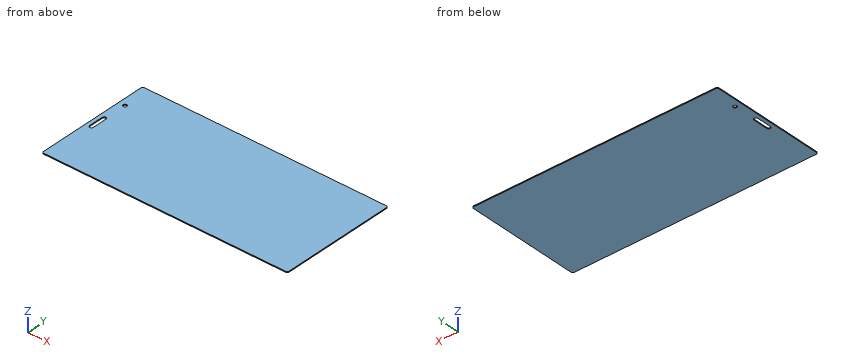
from build123d import *

# Parameters (mm, degrees)
CYLINDER010_R     = 1
CYLINDER010_DEPTH = 10
BOX016_W          = 2
BOX016_H          = 10
BOX016_DEPTH      = 10
FILLET008_R       = 0.95
BOX004_W          = 133
BOX004_H          = 63
BOX004_DEPTH      = 0.5
FILLET005_R       = 1


with BuildPart() as cilindro010:
    # Cylinder010 → Cylinder010 (new body)
    with BuildSketch(Plane(origin=(5.5, 50, 0), x_dir=(1, 0, 0), z_dir=(0, 0, 1))):
        Circle(CYLINDER010_R)
    extrude(amount=CYLINDER010_DEPTH)


with BuildPart() as fillet008:
    # Box016 → Box016 (new body)
    with BuildSketch(Plane(origin=(4, 28.5, 0), x_dir=(1, 0, 0), z_dir=(0, 0, 1))):
        with Locations((1, 5)):
            Rectangle(BOX016_W, BOX016_H)
    extrude(amount=BOX016_DEPTH)

    # Fillet008
    fillet008_edges = [fillet008.edges().sort_by_distance(p)[0] for p in [
        (4, 28.5, 5),
        (4, 38.5, 5),
        (6, 28.5, 5),
        (6, 38.5, 5),
    ]]
    fillet(fillet008_edges, radius=FILLET008_R)


with BuildPart() as cut016:
    # Box004 → Box004 (new body)
    with BuildSketch(Plane(origin=(2, 2, 5.5), x_dir=(1, 0, 0), z_dir=(0, 0, 1))):
        with Locations((66.5, 31.5)):
            Rectangle(BOX004_W, BOX004_H)
    extrude(amount=BOX004_DEPTH)

    # Fillet005
    fillet005_edges = [cut016.edges().sort_by_distance(p)[0] for p in [
        (2, 2, 5.75),
        (2, 65, 5.75),
        (135, 2, 5.75),
        (135, 65, 5.75),
    ]]
    fillet(fillet005_edges, radius=FILLET005_R)


with BuildPart() as cut016_1:
    # Fillet005 placement: moved
    add(cut016.part.moved(Location((0, 0, 1.5))))

    # Cut014: cut Fillet008
    add(fillet008.part, mode=Mode.SUBTRACT)

    # Cut016: cut Cilindro010
    add(cilindro010.part, mode=Mode.SUBTRACT)


solid = cut016_1.part
Could you check a few things on this model? Use its own coordinates, in mm. Coordinates: 2 decimals unless noted, no trailing zeros. Write each loop counter-clockwise with the first axis right and the second up, starting at its lowest first coordinate (ties: lowest second). Pieces come first, ordered by that corner, then holes. Notation, with made-up numbers: M 57.25,10 L 114.25,10 A11 ccw 114.25,14 Z; hole C 86.25,-37.5 d7. An arc over 180 degrees is marked long. One line per question, with ' | ' between items.
1) For pin 1 Ø2.5 at (x, y) = (5.5, 50) entering from +Z, with a flat end and sliding along its axis, tell me the tip position at first contact or that it passes through.
Checks:
pin 1: z = 7.5
2) I need wall thicknesses on probe 1 along X at (y, z) = (33.5, 7.1); probe 2 along X at (y, z) = (50, 7.35); probe 3 along Y at (x, z) = (5.5, 7.2). Which ranges of each line are inside material? Lowest first, please. Write a range as [from, to].
Checks:
probe 1: [2, 4], [6, 135] | probe 2: [2, 4.5], [6.5, 135] | probe 3: [2, 28.61], [38.39, 49], [51, 65]
3) Imagine slicing it at A-A, the plane y = 31.5. Write out the boundary of the cut face in (x, z), and give its area (3 significant figures).
Checks:
outline: M 2,7 L 4,7 L 4,7.5 L 2,7.5 Z; M 6,7 L 135,7 L 135,7.5 L 6,7.5 Z | area: 65.5 mm²
